Can you work these out from the model? Positions are in its coordinate system, mm. A direction names the side the tool comes from. Round coordinates to 2 decimals unless told otherwise and drop trailing zeros. Loops run counter-clockwise (first coordinate to the right, second up) from the corner with the lowest first, then second, coordinate; pieces in that order, holes last.
(1) I want a section at A-A on z = 1.7. Write out the boundary of the cut face in (x, y), plus the area to 3 significant figures.
(2) Thinking about a two-plate mould opening in X: for faces 1 (the face through (-38, 138, 5)), 2 (the face through (35.2, 127.65, 2.46)), 3 (the face through (-41, 178, 2)), which applies, released by +X, released by -X, zero draft, split by the parting line, or undercut?
(3) I want a section at B-B on y = 86.5. Write out the boundary of the cut face in (x, z), plus the area to 3 significant figures.
(4) Which directions (+Z, -Z, +X, -X, +Y, -Y) give clear straight access to the entire face, cutting with the end or side of a thin tool? Please do faces 4 (the face through (12.36, 140.4, 2.46)), 5 (the face through (42.24, 133.79, 2.46)).
(5) If I drill on line 1 along X through (y, z) = (137, 4.65); line 2 along X through (y, z) = (135.5, 4.75); line 3 along X through (y, z) = (118.5, 3.75), over which ranges is the centre line in solid material (lowest first)?
(6) I want a section at C-C on x = -86. Write out the boundary of the cut face in (y, z), plus the area to 3 significant figures.
(7) Will these pins go through, and if not, where does the flat tip stop? pin 1 Ø6 at (x, y) = (-9.5, 156.5) entering from -Z; pin 2 Ø2 at (x, z) = (-81.5, 3) entering from +Y; pin 3 Ø2 at (y, z) = (126, 4.5) entering from -X.
from build123d import *

# Parameters (mm, degrees)
SKETCH1_R           = 1.25
BOSS_EXTRUDE1_DEPTH = 5


with BuildPart() as part:
    # Sketch1 → Boss-Extrude1 (new body)
    with BuildSketch(Plane.XY):
        with BuildLine():
            Line((-14.530655618, 146.054710198), (-14.530655618, 76.440036381))
            ThreePointArc((-14.530655618, 76.440036381), (-16.050878115, 74.140028546), (-18.762684454, 74.637239634))
            ThreePointArc((-18.762684454, 74.637239634), (-39.533713803, 83.001706864), (-60.309436884, 74.648904776))
            ThreePointArc((-60.309436884, 74.648904776), (-63.02087634, 74.152941195), (-64.540453099, 76.452673847))
            Line((-64.540453099, 76.452673847), (-64.540453099, 146.054594281))
            ThreePointArc((-64.540453099, 146.054594281), (-65.483745675, 148.010779854), (-67.601782697, 148.490761164))
            ThreePointArc((-67.601782697, 148.490761164), (-91.160542777, 140.523686318), (-112.675804189, 128.050395473))
            ThreePointArc((-112.675804189, 128.050395473), (-114.338855979, 127.585787298), (-115.90638117, 128.309988089))
            Line((-115.90638117, 128.309988089), (-126.685409475, 139.089016395))
            ThreePointArc((-126.685409475, 139.089016395), (-127.417578865, 140.874623829), (-126.659999819, 142.649599861))
            ThreePointArc((-126.659999819, 142.649599861), (-39.537255282, 178.008774119), (47.582728327, 142.642797871))
            ThreePointArc((47.582728327, 142.642797871), (48.340215149, 140.859037128), (47.595476063, 139.069916571))
            Line((47.595476063, 139.069916571), (36.734698992, 128.361391788))
            ThreePointArc((36.734698992, 128.361391788), (35.171966674, 127.649015862), (33.518380328, 128.112981328))
            ThreePointArc((33.518380328, 128.112981328), (12.04095694, 140.545885375), (-11.469336287, 148.490879447))
            ThreePointArc((-11.469336287, 148.490879447), (-13.587367163, 148.010892491), (-14.530655618, 146.054710198))
        make_face()
        with Locations((-110.157771622, 143.774581978)):
            Circle(SKETCH1_R, mode=Mode.SUBTRACT)
        with Locations((31.073501699, 143.774581978)):
            Circle(SKETCH1_R, mode=Mode.SUBTRACT)
        with Locations((-39.71763232, 92.992417004)):
            Circle(SKETCH1_R, mode=Mode.SUBTRACT)
    extrude(amount=BOSS_EXTRUDE1_DEPTH)


solid = part.part
Filled sheet:
1. outline: (-126.69, 139.09) - (-115.91, 128.31) arc R2.5 ccw to (-112.68, 128.05) arc R125 cw to (-67.6, 148.49) arc R2.5 cw to (-64.54, 146.05) - (-64.54, 76.45) arc R2.5 ccw to (-60.31, 74.65) arc R29.99 cw to (-18.76, 74.64) arc R2.5 ccw to (-14.53, 76.44) - (-14.53, 146.05) arc R2.5 cw to (-11.47, 148.49) arc R125 cw to (33.52, 128.11) arc R2.5 ccw to (36.73, 128.36) - (47.6, 139.07) arc R2.5 ccw to (47.58, 142.64) arc R125 ccw to (-126.66, 142.65) arc R2.5 ccw to start; hole circle Ø2.5 at (-110.16, 143.77); hole circle Ø2.5 at (-39.72, 92.99); hole circle Ø2.5 at (31.07, 143.77)
1. area: 7,880 mm2
2. face 1: zero draft
2. face 2: undercut
2. face 3: split by the parting line
3. outline: (-64.54, 0) - (-14.53, 0) - (-14.53, 5) - (-64.54, 5) - close
3. area: 250 mm2
4. face 4: +Z, -Z, -Y
4. face 5: +Z, -Z, +X, -Y
5. line 1: x = -124.6 to -98.31, -64.54 to -14.53, 19.24 to 45.5
5. line 2: x = -123.1 to -101.05, -64.54 to -14.53, 21.98 to 43.97
5. line 3: x = -64.54 to -14.53
6. outline: (142.73, 0) - (169.05, 0) - (169.05, 5) - (142.73, 5) - close
6. area: 132 mm2
7. pin 1: stops at z = 0
7. pin 2: stops at y = 171.11
7. pin 3: stops at x = -64.54
